Part print with two shaded views. Sizes in mm from the minimum x, y, z corner. Give positions to 0.01 mm unless a question says otherwise; leave off trailing zeros. Loops run counter-clockwise (first coordinate to the right, second up) from the corner with the lowest first, then second, coordinate; pieces in that order, holes last. Notation, with made-up numbers: M -31,24 L -11,24 A21 cw -11,39 Z; hole C -7.5,21.5 d4. An arc over 180 degrees is marked long. Answer as a JSON object with one key per item and string values. Group by question number.
1. Slice it at D-D (x = 11). List the corners of the cut face in (y, z).
2. Drill centre lines: line 1 along Y through (x, z) = (129.5, 19); line 2 along X through (y, z) = (18.5, 24.75) (1 decimal); line 3 along Y through (x, z) = (168, 16). Where is each one in solid material? Low to high. Write a range as [from, to].
3. Mould opens along Y. For the marked faces 1, 2 and 3 say: released by +Y, released by -Y, zero draft, split by the parting line, or undercut.
4. Slice it at C-C (z = 8). List the corners of the cut face in (x, y) (1 decimal), then the cut area to 3 significant figures.
5. Slice it at A-A (y = 12.5). List the corners of the cut face in (x, z) (1 decimal).
6. Slice it at B-B (x = 129). List the corners of the cut face in (y, z), then the cut area to 3 significant figures.
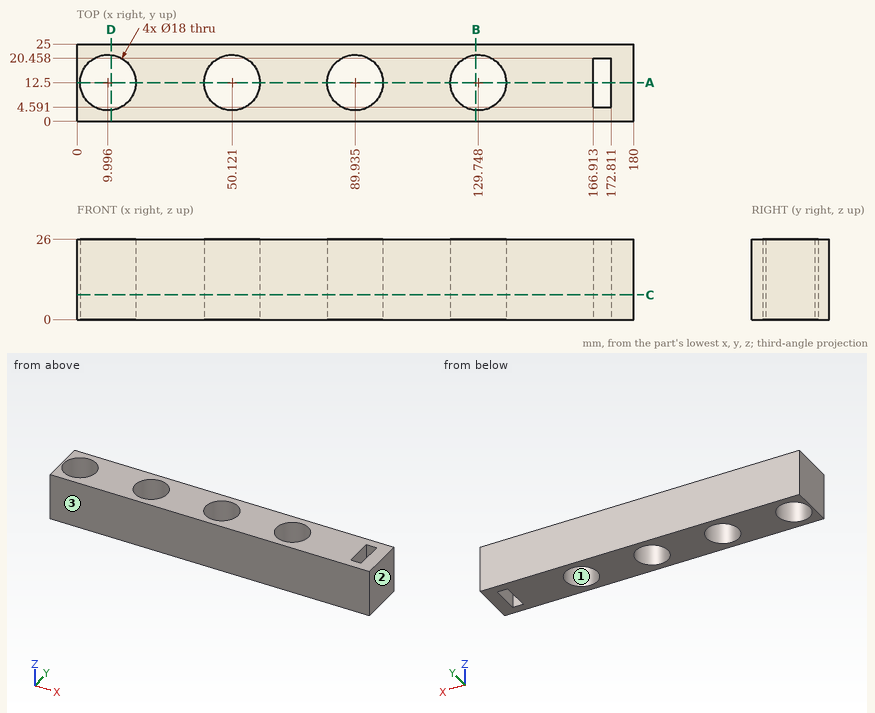
Established:
{
 "1": {"outline": "M 0,0 L 3.56,0 L 3.56,26 L 0,26 Z; M 21.44,0 L 25,0 L 25,26 L 21.44,26 Z"},
 "2": {"line 1": "y = [0, 3.5], [21.5, 25]", "line 2": "x = [0, 3.3], [16.7, 43.4], [56.8, 83.2], [96.6, 123], [136.5, 166.9], [172.8, 180]", "line 3": "y = [0, 4.59], [20.46, 25]"},
 "3": {"face 1": "undercut", "face 2": "zero draft", "face 3": "released by -Y"},
 "4": {"outline": "M 0,0 L 180,0 L 180,25 L 0,25 Z; hole C 10,12.5 d18; hole C 50.1,12.5 d18; hole C 89.9,12.5 d18; hole C 129.7,12.5 d18; hole M 166.9,4.6 L 172.8,4.6 L 172.8,20.5 L 166.9,20.5 Z", "area": "3,390 mm^2"},
 "5": {"outline": "M 0,0 L 1,0 L 1,26 L 0,26 Z; M 19,0 L 41.1,0 L 41.1,26 L 19,26 Z; M 59.1,0 L 80.9,0 L 80.9,26 L 59.1,26 Z; M 98.9,0 L 120.7,0 L 120.7,26 L 98.9,26 Z; M 138.7,0 L 166.9,0 L 166.9,26 L 138.7,26 Z; M 172.8,0 L 180,0 L 180,26 L 172.8,26 Z"},
 "6": {"outline": "M 0,0 L 3.53,0 L 3.53,26 L 0,26 Z; M 21.47,0 L 25,0 L 25,26 L 21.47,26 Z", "area": "184 mm^2"}
}
